Can you work these out from the model? Positions are in its coordinate system, mm. Face numbers are marked on the shaded views. A direction names the side the tool comes from. Round coordinates to 2 decimals unless told otherwise and drop trailing zeros. Loops run counter-clockwise (first coordinate to the right, second up) from the corner with the lowest first, then second, coordinate; pieces in that order, holes last. Notation, with made-up numbers: M -11.75,46 L 5.25,46 A13 ccw 5.25,58 Z; hole C -16,-34 d11. An arc over 180 degrees is marked long. Return JSON: item names as keys, results as strings.
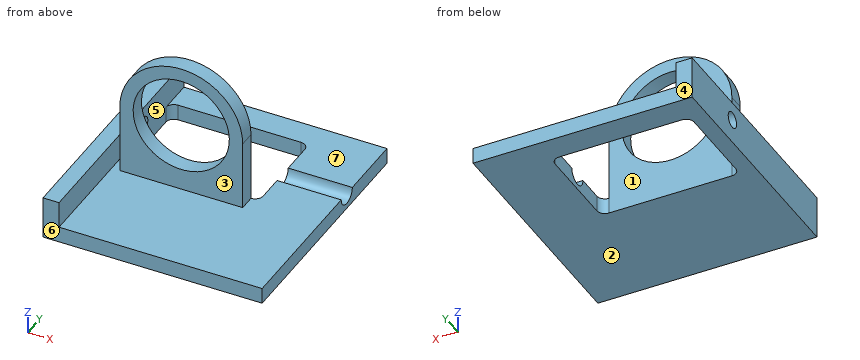
```python
from build123d import *

# Parameters (mm, degrees)
SKETCH1_W           = 41
SKETCH1_H           = 45
BOSS_EXTRUDE1_DEPTH = 3
SKETCH2_W           = 5
SKETCH2_H           = 45
SKETCH2_R           = 1.5
BOSS_EXTRUDE2_DEPTH = 3
SKETCH4_R           = 9
BOSS_EXTRUDE3_DEPTH = 3
CUT_EXTRUDE4_DEPTH  = 12


with BuildPart() as part:
    # Sketch1 → Boss-Extrude1 (new body)
    with BuildSketch(Plane.XY):
        with Locations((20.5, -22.5)):
            Rectangle(SKETCH1_W, SKETCH1_H)
        with BuildLine():
            Line((27.5, -23), (4.5, -23))
            ThreePointArc((4.5, -23), (3.439339828, -22.560660172), (3, -21.5))
            Line((3, -21.5), (3, -6.5))
            ThreePointArc((3, -6.5), (3.439339828, -5.439339828), (4.5, -5))
            Line((4.5, -5), (27.5, -5))
            ThreePointArc((27.5, -5), (28.560660172, -5.439339828), (29, -6.5))
            Line((29, -6.5), (29, -21.5))
            ThreePointArc((29, -21.5), (28.560660172, -22.560660172), (27.5, -23))
        make_face(mode=Mode.SUBTRACT)
    extrude(amount=BOSS_EXTRUDE1_DEPTH)

    # Sketch2 → Boss-Extrude2 (add)
    with BuildSketch(Plane(origin=(0, 0, 0), x_dir=(0, 0, -1), z_dir=(1, 0, 0))):
        with Locations((-5.5, -22.5)):
            Rectangle(SKETCH2_W, SKETCH2_H)
        with Locations((-4.51, -14.5)):
            Circle(SKETCH2_R, mode=Mode.SUBTRACT)
    extrude(amount=BOSS_EXTRUDE2_DEPTH)

    # Sketch4 → Boss-Extrude3 (add)
    with BuildSketch(Plane(origin=(0, -23, 0), x_dir=(1, 0, 0), z_dir=(0, 1, 0))):
        with BuildLine():
            Line((4.5, -3), (4.5, -16))
            ThreePointArc((4.5, -16), (16, -27.5), (27.5, -16))
            Line((27.5, -16), (27.5, -3))
            Line((27.5, -3), (4.5, -3))
        make_face()
        with Locations(Location((16, -16, 0), (0, 0, 270))):
            Circle(SKETCH4_R, mode=Mode.SUBTRACT)
    extrude(amount=-BOSS_EXTRUDE3_DEPTH)

    # Sketch7 → Cut-Extrude4 (cut)
    with BuildSketch(Plane(origin=(41, 0, 0), x_dir=(0, 0, -1), z_dir=(1, 0, 0))):
        with BuildLine():
            Line((-3, -12.5), (-3, -16.5))
            ThreePointArc((-3, -16.5), (-1, -14.5), (-3, -12.5))
        make_face()
    extrude(amount=-CUT_EXTRUDE4_DEPTH, mode=Mode.SUBTRACT)


solid = part.part
```
Q1. On a 3-axis mill with a long thin cutter (end or side, diameter ignored), from which of +Z, -Z, +X, -X, +Y, -Y can I reach the whole of each face in a straight line? I mean the marked faces 5, 6 and 7. Say none if no direction works.
Results:
{"face 5": "+Z", "face 6": "+Z, -Z, +X, -X, -Y", "face 7": "+Z, +X, +Y"}
Q2. Suppose I cut it at B-B, the plane y = -24. Please give me the cut outline in (x, z), plus the area to 3 significant figures.
Results:
{"outline": "M 0,0 L 41,0 L 41,3 L 27.5,3 L 27.5,16 A11.5 ccw 4.5,16 L 4.5,3 L 3,3 L 3,8 L 0,8 Z; hole C 16,16 d18", "area": "390 mm2"}
Q3. If I drill on line 1 along X through (y, z) = (-24.25, 16); line 2 along Y through (x, z) = (11.5, 2.5); line 3 along Y through (x, z) = (0.7, 4.51), over which ranges is the centre line in solid material (lowest first)?
Results:
{"line 1": "x = 4.5 to 7, 25 to 27.5", "line 2": "y = -45 to -23, -5 to 0", "line 3": "y = -45 to -16, -13 to 0"}
Q4. Thinking about a two-plate mould opening in Y: for the marked faces 1, 2, 3 and 4, which applies, pulls with the +Y half, pulls with the -Y half, needs draft (parallel to the pull), parting line crosses it, or undercut?
Results:
{"face 1": "undercut", "face 2": "needs draft", "face 3": "pulls with the -Y half", "face 4": "pulls with the +Y half"}
Q5. I'm going to push flat-ended pins straight in: pin 1 Ø3.5 at (y, z) = (-24, 11.5) entering from +X; pin 2 Ø1.5 at (y, z) = (-25, 12) entering from -X; pin 3 Ø14 at (x, y) = (14, -5) entering from +Z. Where does each tip first touch, or does it pass through?
Results:
{"pin 1": "stops at x = 27.5", "pin 2": "stops at x = 4.5", "pin 3": "stops at z = 3"}
Q6. Suppose I cut it at C-C, the plane x = 16. Please give me the cut outline in (y, z), plus the area to 4 significant figures.
Results:
{"outline": "M -45,0 L -23,0 L -23,7 L -26,7 L -26,3 L -45,3 Z; M -26,25 L -23,25 L -23,27.5 L -26,27.5 Z; M -5,0 L 0,0 L 0,3 L -5,3 Z", "area": "100.5 mm2"}
Q7. Suppose I cut it at D-D, the plane y = -30. Please give me the cut outline in (x, z).
Results:
{"outline": "M 0,0 L 41,0 L 41,3 L 3,3 L 3,8 L 0,8 Z"}
Q8. Suppose I cut it at A-A, the plane z = 4.51. Please give me the cut outline in (x, y), plus the area to 3 significant figures.
Results:
{"outline": "M 0,-45 L 3,-45 L 3,-16 L 0,-16 Z; M 0,-13 L 3,-13 L 3,0 L 0,0 Z; M 4.5,-26 L 27.5,-26 L 27.5,-23 L 4.5,-23 Z", "area": "195 mm2"}
